```python
from build123d import *

# Parameters (mm, degrees)
ESQUISSE1_W        = 110
ESQUISSE1_H        = 71
ESQUISSE1_R        = 1.75
BOSS_EXTRU_1_DEPTH = 6
CONG_1_R           = 5


with BuildPart() as part:
    # Esquisse1 → Boss.-Extru.1 (new body)
    with BuildSketch(Plane.XY):
        Rectangle(ESQUISSE1_W, ESQUISSE1_H)
        with Locations((-50, 30.5)):
            Circle(ESQUISSE1_R, mode=Mode.SUBTRACT)
        with Locations((50, 30.5)):
            Circle(ESQUISSE1_R, mode=Mode.SUBTRACT)
        with Locations((50, -30.5)):
            Circle(ESQUISSE1_R, mode=Mode.SUBTRACT)
        with Locations((-50, -30.5)):
            Circle(ESQUISSE1_R, mode=Mode.SUBTRACT)
        with Locations((-50, 0)):
            Circle(ESQUISSE1_R, mode=Mode.SUBTRACT)
        with Locations((50, 0)):
            Circle(ESQUISSE1_R, mode=Mode.SUBTRACT)
    extrude(amount=BOSS_EXTRU_1_DEPTH)

    # Congé1
    cong_1_edges = [part.edges().sort_by_distance(p)[0] for p in [
        (-55, 35.5, 3),
        (55, 35.5, 3),
        (55, -35.5, 3),
        (-55, -35.5, 3),
    ]]
    fillet(cong_1_edges, radius=CONG_1_R)


solid = part.part
```
Read the model definition and answer for the solid it produces. Units are mm, in the model's axes. Give positions to 0.01 mm unless a question says otherwise; leave off trailing zeros. Write item = value, one per line. Start each with the question number.
Item 1: Find the intervals of material crossed by probe 1 along Y at (x, z) = (50, 2.1), in increasing order. Write a range as [from, to].
Item 2: The mould has two halves that part along X. Classify faces 1 (the cylindrical face through (53.5, 34.07, 3.04)), 2 (the cylindrical face through (-48.383, -0.67, 2.958)), 3 (the cylindrical face through (-53.57, -34, 3.04)), 4 (the flat face through (-1, 0, 0)): +X half, -X half, draft (parallel to the pull), parting line (faces both ways), or undercut.
Item 3: Each of these flat-tipped pins is pushed along its axis until it touches: P1, Ø4.5, axis at x = -50, y = -30.5, coming from the +Z side; P2, Ø2, axis at x = 50, y = -30.5, coming from the -Z side. Where does it stop, or does it pass through?
Response:
q1.probe_1 = [-35.5, -32.25], [-28.75, -1.75], [1.75, 28.75], [32.25, 35.5]
q2.face_1 = +X half
q2.face_2 = undercut
q2.face_3 = -X half
q2.face_4 = draft
q3.P1 = 6
q3.P2 = through
